The listing builds one solid part. Answer for the finished solid, in the listing's coordinates (mm). A direction names the side the tool comes from. Round coordinates to 2 decimals unless told otherwise and drop trailing zeros. Loops run counter-clockwise (first coordinate to the right, second up) from the corner with the lowest first, then second, coordinate; pieces in that order, holes last. Notation, with made-up numbers: (29.5, -6.5) - (60.5, -6.5) arc R14 cw to (60.5, 11.5) - close; hole circle Ø4 at (60.25, 51). An arc over 180 degrees is marked (long way). One line per item, written item: value.
```python
from build123d import *

# Parameters (mm, degrees)
BOSS_EXTRUDE1_DEPTH = 2.5
SKETCH2_R           = 1.78
CUT_EXTRUDE1_DEPTH  = 1.5
FILLET1_R           = 1.5


with BuildPart() as part:
    # Sketch1 → Boss-Extrude1 (new body)
    with BuildSketch(Plane(origin=(0, 0, 0), x_dir=(1, 0, 0), z_dir=(0, 1, 0))):
        Polygon((-21.216153836, 11.741903429), (-21.216153836, 8.241903429), (-8.120509951, -0.958096571), (-4.216153836, -0.958096571), (-4.216153836, 11.741903429), align=None)
    extrude(amount=BOSS_EXTRUDE1_DEPTH)

    # Sketch2 → Cut-Extrude1 (cut)
    with BuildSketch(Plane(origin=(0, 2.5, 0), x_dir=(1, 0, 0), z_dir=(0, 1, 0))):
        with Locations((-17.966153836, 8.241903429)):
            Circle(SKETCH2_R)
    extrude(amount=-CUT_EXTRUDE1_DEPTH, mode=Mode.SUBTRACT)

    # Fillet1
    fillet1_edges = [part.edges().sort_by_distance(p)[0] for p in [
        (-6.168331894, 0, 0.958096571),
        (-14.668331894, 0, -3.641903429),
        (-21.216153836, 0, -9.991903429),
        (-12.716153836, 0, -11.741903429),
        (-8.120509951, 1.25, 0.958096571),
        (-21.216153836, 1.25, -8.241903429),
        (-21.216153836, 1.25, -11.741903429),
    ]]
    fillet(fillet1_edges, radius=FILLET1_R)

    # Mirror1: part across plane


with BuildPart() as part_1:
    add(part.part)
    add(part.part.mirror(Plane(origin=(-4.216153836, 2.5, 0.958096571), x_dir=(0, 0, 1), z_dir=(-1, 0, 0))))


solid = part_1.part
```
1) For a pull along Z with two mould halves and no side action, classify faces 3 (the flat face through (-14.628, 1.993, -3.614)), 4 (the cylindrical face through (-20.79, 2.01, -11.29)), 5 (the flat face through (-4, 0, -7)), 6 (the cylindrical face through (9.8, 1.8, -10)) as released by +Z, released by -Z, zero draft, split by the parting line, or undercut.
Final values:
face 3: released by +Z
face 4: released by -Z
face 5: zero draft
face 6: undercut
2) A cutting plane is placed at A-A on y = 1.95. Give the vertices of the cut face in (x, z), and give its area (3 significant figures).
Final values:
outline: (-21.22, -10.24) arc R1.5 ccw to (-19.72, -11.74) - (11.28, -11.74) arc R1.5 ccw to (12.78, -10.24) - (12.78, -9.02) arc R1.5 ccw to (12.15, -7.79) - (0.08, 0.69) arc R1.5 ccw to (-0.79, 0.96) - (-7.65, 0.96) arc R1.5 ccw to (-8.51, 0.69) - (-20.58, -7.79) arc R1.5 ccw to (-21.22, -9.02) - close; hole circle Ø3.56 at (-17.97, -8.24); hole circle Ø3.56 at (9.53, -8.24)
area: 290 mm2
3) For faces 1 (the cylindrical face through (-20.79, 0.45, -9.62)), 2 (the flat face through (-18, 1, -8)), determine the directions among +Z, -Z, +X, -X, +Y, -Y from which every point of the face is accessible in a straight line to the end or side of a thin tool.
Final values:
face 1: +Z, -Z, -X, -Y
face 2: +Y
4) Consider L1, parallel to X at y = 2.25, z = -8.25; L2, parallel to X at y = 1.3, z = -7.5; L3, parallel to Y at x = 10, z = -9.75. Determine where each line is inside the solid, lowest interval first.
Final values:
L1: -21 to -19.75, -16.19 to 7.75, 11.31 to 12.57
L2: -20.14 to -19.58, -16.35 to 7.92, 11.15 to 11.7
L3: 0 to 1
5) A cutting plane is placed at B-B on x = -5. Give the vertices of the cut face in (y, z).
Final values:
outline: (0, -10.24) arc R1.5 ccw to (1.5, -11.74) - (2.5, -11.74) - (2.5, 0.96) - (1.5, 0.96) arc R1.5 ccw to (0, -0.54) - close
6) A cutting plane is placed at C-C on y = 0.55. Give the vertices of the cut face in (x, z), and give its area (3 significant figures).
Final values:
outline: (-20.88, -10.24) arc R1.16 ccw to (-19.72, -11.4) - (11.28, -11.4) arc R1.16 ccw to (12.44, -10.24) - (12.44, -9.02) arc R1.16 ccw to (11.95, -8.07) - (-0.12, 0.41) arc R1.16 ccw to (-0.79, 0.62) - (-7.65, 0.62) arc R1.16 ccw to (-8.31, 0.41) - (-20.38, -8.07) arc R1.16 ccw to (-20.88, -9.02) - close
area: 284 mm2
7) This flat-tipped pin is pushed along its axis until it touches: pin 1 Ø1.1 at (x, z) = (10, -7.5) entering from +Y. Where does it stop, or does it pass through?
Final values:
pin 1: y = 1
